from build123d import *

# Parameters (mm, degrees)
BOSS_EXTRUDE2_DEPTH = 22.86
CUT_EXTRUDE1_DEPTH  = 23.8600001
SKETCH10_R          = 3.96875
CUT_EXTRUDE2_DEPTH  = 23.8600001
BOSS_EXTRUDE4_DEPTH = 22.86
SKETCH13_R          = 3.96875
CUT_EXTRUDE5_DEPTH  = 23.8600001
LPATTERN1_COUNT     = 2
LPATTERN1_PITCH     = 64
SKETCH14_R          = 2.54
CUT_EXTRUDE6_DEPTH  = 23.8600001
SKETCH15_R          = 3.96875
CUT_EXTRUDE7_DEPTH  = 23.8600001
SKETCH16_R          = 3.96875
CUT_EXTRUDE8_DEPTH  = 23.8600001
SKETCH19_R          = 3.96875
CUT_EXTRUDE11_DEPTH = 23.8600001
SKETCH21_R          = 2.54
CUT_EXTRUDE12_DEPTH = 23.8600001
SKETCH23_R          = 4.16785984
SKETCH23_R_2        = 4.440390953
BOSS_EXTRUDE5_DEPTH = 22.86
CUT_EXTRUDE13_DEPTH = 23.8600001
FILLET1_R           = 3.175


with BuildPart() as part:
    # Sketch6 → Boss-Extrude2 (new body)
    with BuildSketch(Plane.XY):
        with BuildLine():
            Line((-68.006850091, -76.67090114), (-109.486767671, -48.656527855))
            Line((-109.486767671, -48.656527855), (-118.371760678, -61.812230963))
            Line((-118.371760678, -61.812230963), (18.447551645, -154.216158235))
            Line((18.447551645, -154.216158235), (135.729459338, 19.43912279))
            Line((135.729459338, 19.43912279), (-1.089852986, 111.843050063))
            Line((-1.089852986, 111.843050063), (-73.946795643, 3.966284577))
            Line((-73.946795643, 3.966284577), (-56.624438948, -7.732749433))
            ThreePointArc((-56.624438948, -7.732749433), (-43.058385537, 37.577891571), (0, 57.15))
            ThreePointArc((0, 57.15), (56.404848571, 31.095576642), (70.829334649, -29.338471048))
            add(Edge.make_bspline(
                [(70.829334649, -29.338471048), (70.811686062, -29.418295928), (70.776015112, -29.578104383), (70.713320217, -29.85478305), (70.619021771, -30.262929245), (70.501052001, -30.762086912), (70.364034474, -31.322191481), (70.199318515, -31.970958926), (70.000453855, -32.723919765), (69.795103485, -33.469783355), (69.582015398, -34.214296028), (69.361377803, -34.956693289), (69.133257682, -35.696762218), (68.838782679, -36.61892651), (68.470566207, -37.720710028), (68.019498024, -38.998776477), (67.474836154, -40.448808619), (66.901337925, -41.887676852), (66.299328392, -43.31485223), (65.669141732, -44.729810424), (65.011119088, -46.132040323), (64.325609411, -47.52103904), (63.612968547, -48.896314904), (62.87355937, -50.257385735), (62.107751613, -51.603779381), (61.315921169, -52.935034173), (60.49845004, -54.250698756), (59.655726138, -55.550331897), (58.571247582, -57.154294757), (57.220953058, -59.045283389), (55.576035723, -61.200397094), (53.604026134, -63.590264702), (51.54329346, -65.904053004), (49.39728314, -68.138962994), (47.169496434, -70.29235602), (44.863486103, -72.361752995), (42.482847363, -74.344831806), (40.031215607, -76.239428526), (36.882516177, -78.494556171), (32.976808929, -81.016011003), (28.250788286, -83.68089187), (21.41551215, -86.919136497), (14.30829026, -89.526654921), (6.996956895, -91.488176442), (-0.451922312, -92.797413176), (-6.61686174, -93.456358442), (-12.81195397, -93.702029749), (-19.009644204, -93.537285056), (-25.183124422, -92.966685286), (-31.306438312, -91.996382122), (-36.598524037, -90.804323442), (-41.072542301, -89.543185606), (-44.752319298, -88.33589156), (-47.664184976, -87.27761875), (-50.541347258, -86.128353728), (-53.381128552, -84.889612663), (-56.180924218, -83.562977818), (-58.593536599, -82.326710176), (-60.633378351, -81.214215821), (-62.313751085, -80.252471782), (-63.646071553, -79.462491566), (-64.966093336, -78.652178853), (-66.222359154, -77.854259082), (-67.143044791, -77.250601571), (-67.736251212, -76.85365602), (-68.006850091, -76.67090114)],
                knots=[0.071020771, 0.071020771, 0.071020771, 0.071020771, 0.071020771, 0.072848477, 0.074676184, 0.07650389, 0.078331597, 0.08198701, 0.085642423, 0.089297836, 0.092953249, 0.096608662, 0.100264075, 0.103919488, 0.107574901, 0.114885727, 0.122196554, 0.12950738, 0.136818214, 0.144129048, 0.151439882, 0.158750716, 0.166061558, 0.173372401, 0.180683243, 0.187994085, 0.195304924, 0.202615763, 0.209926602, 0.217237441, 0.231859103, 0.246480766, 0.261102426, 0.275724085, 0.290345754, 0.304967424, 0.319589099, 0.334210774, 0.348832457, 0.36345414, 0.392697464, 0.421940789, 0.451184112, 0.506140643, 0.535383973, 0.564627303, 0.593870641, 0.623113979, 0.652357319, 0.68160066, 0.710843985, 0.740087309, 0.754708984, 0.769330659, 0.783952333, 0.798574008, 0.813195669, 0.82781733, 0.842438991, 0.849749821, 0.857060652, 0.86437149, 0.871682327, 0.878993165, 0.885158103, 0.885158103, 0.885158103, 0.885158103, 0.885158103], degree=4))
        make_face()
    extrude(amount=BOSS_EXTRUDE2_DEPTH)

    # Sketch8 → Cut-Extrude1 (cut, through all)
    with BuildSketch(Plane.XY.offset(22.86)):
        Polygon((-71.011229489, -93.798205788), (-53.378672597, -90.381637707), (-42.854110111, -97.489632113), (-39.43754203, -115.122189004), align=None)
    extrude(amount=-CUT_EXTRUDE1_DEPTH, mode=Mode.SUBTRACT)

    # Sketch10 → Cut-Extrude2 (cut, through all)
    with BuildSketch(Plane.XY.offset(22.86)):
        with Locations((4.996496209, -84.796642912)):
            Circle(SKETCH10_R)
        with Locations((40.816310536, -31.759477627)):
            Circle(SKETCH10_R)
        with Locations((76.636124864, 21.277687659)):
            Circle(SKETCH10_R)
        with Locations((-45.295165913, -45.214466102)):
            Circle(SKETCH10_R)
    extrude(amount=-CUT_EXTRUDE2_DEPTH, mode=Mode.SUBTRACT)

    # Sketch12 → Boss-Extrude4 (add, through all)
    with BuildSketch(Plane.XY.offset(22.86)):
        Polygon((135.729459338, 19.43912279), (67.319803176, 65.641086427), (88.643786393, 97.214773886), (157.053442554, 51.01281025), align=None)
    extrude(amount=-BOSS_EXTRUDE4_DEPTH)

    # Sketch13 → Cut-Extrude5 (cut, through all)
    with BuildSketch(Plane.XY.offset(22.86)):
        with Locations((94.899221836, -29.671127724)):
            Circle(SKETCH13_R)
    cut_extrude5 = extrude(amount=-CUT_EXTRUDE5_DEPTH, mode=Mode.SUBTRACT)

    # LPattern1: Cut-Extrude5 ×2
    with Locations(*[Vector(-0.559684599, -0.828705708, 0) * (i * LPATTERN1_PITCH) for i in range(1, LPATTERN1_COUNT)]):
        add(cut_extrude5, mode=Mode.SUBTRACT)

    # Sketch14 → Cut-Extrude6 (cut, through all)
    with BuildSketch(Plane.XY.offset(22.86)):
        with Locations((71.72703343, -52.635713164)):
            Circle(SKETCH14_R)
        with Locations((35.907219102, -105.67287845)):
            Circle(SKETCH14_R)
        with Locations((115.740620068, 63.589229581)):
            Circle(SKETCH14_R)
    extrude(amount=-CUT_EXTRUDE6_DEPTH, mode=Mode.SUBTRACT)

    # Sketch15 → Cut-Extrude7 (cut, through all)
    with BuildSketch(Plane.XY.offset(22.86)):
        with Locations((-105.147343009, -59.249804902)):
            Circle(SKETCH15_R)
        with Locations((15.885125585, -140.991740566)):
            Circle(SKETCH15_R)
        with Locations((1.472573075, 98.618632394)):
            Circle(SKETCH15_R)
    extrude(amount=-CUT_EXTRUDE7_DEPTH, mode=Mode.SUBTRACT)

    # Sketch16 → Cut-Extrude8 (cut, through all)
    with BuildSketch(Plane.XY.offset(22.86)):
        with Locations((92.060354474, 79.582216994)):
            Circle(SKETCH16_R)
        with Locations((139.420885662, 47.596242169)):
            Circle(SKETCH16_R)
    extrude(amount=-CUT_EXTRUDE8_DEPTH, mode=Mode.SUBTRACT)

    # Sketch19 → Cut-Extrude11 (cut, through all)
    with BuildSketch(Plane.XY.offset(22.86)):
        with Locations((-65.680233685, -85.904783923)):
            Circle(SKETCH19_R)
    extrude(amount=-CUT_EXTRUDE11_DEPTH, mode=Mode.SUBTRACT)

    # Sketch21 → Cut-Extrude12 (cut, through all)
    with BuildSketch(Plane.XY.offset(22.86)):
        with Locations((-13.666272317, 70.530227577)):
            Circle(SKETCH21_R)
        with Locations((26.00698069, 78.217505758)):
            Circle(SKETCH21_R)
        with Locations((-86.729358658, -71.688795112)):
            Circle(SKETCH21_R)
        with Locations((-8.64928203, -120.590613931)):
            Circle(SKETCH21_R)
    extrude(amount=-CUT_EXTRUDE12_DEPTH, mode=Mode.SUBTRACT)

    # Sketch23 → Boss-Extrude5 (add, through all)
    with BuildSketch(Plane.XY.offset(22.86)):
        with Locations((-65.680233685, -85.904783923)):
            Circle(SKETCH23_R)
        with Locations((-86.729358658, -71.688795112)):
            Circle(SKETCH23_R_2)
    extrude(amount=-BOSS_EXTRUDE5_DEPTH)

    # Sketch25 → Cut-Extrude13 (cut, through all)
    with BuildSketch(Plane.XY.offset(22.86)):
        Polygon((85.800588631, 93.004948891), (87.167215863, 85.951926135), (71.529628171, 62.797888664), (67.319803176, 65.641086427), align=None)
    extrude(amount=-CUT_EXTRUDE13_DEPTH, mode=Mode.SUBTRACT)

    # Fillet1
    fillet1_edges = [part.edges().sort_by_distance(p)[0] for p in [
        (-73.946795643, 3.966284577, 11.43),
        (-1.089852986, 111.843050063, 11.43),
        (18.447551645, -154.216158235, 11.43),
        (-118.371760678, -61.812230963, 11.43),
        (-109.486767671, -48.656527855, 11.43),
        (85.800588631, 93.004948891, 11.43),
        (87.167215863, 85.951926135, 11.43),
        (71.529628171, 62.797888664, 11.43),
        (-39.43754203, -115.122189004, 11.43),
        (-71.011229489, -93.798205788, 11.43),
        (-53.378672597, -90.381637707, 11.43),
        (-42.854110111, -97.489632113, 11.43),
        (157.053442554, 51.01281025, 11.43),
        (88.643786393, 97.214773886, 11.43),
    ]]
    fillet(fillet1_edges, radius=FILLET1_R)


solid = part.part
Verification items for the finished model (mm, model axes). A direction names the side the tool comes from. Round coordinates to 2 decimals unless told otherwise and drop trailing zeros. Loops run counter-clockwise (first coordinate to the right, second up) from the corner with the lowest first, then second, coordinate; pieces in that order, holes last. Notation, with made-up numbers: (63, -10.75) - (99, -10.75) arc R23 ccw to (99, 21.25) - close; hole circle Ø7 at (-14.75, 19). An arc over 180 degrees is marked (long way). Answer in a Markdown table with one row per item. Add a question column.
Q1. Section check A-A on z = 5. State how many separate pieces and enclosed holes the cut face has, plus the area to 3 significant figures.
Q2. Material ranges on line 1 (Y direction, x = 17.5, z = 17.75); line 2 (Y direction, x = 37, z = 17.25); line 3 (X direction, y = -58, z = 4), recorded low to high.
Q3. Tool access check on faces 1 (the face through (-37.033, 58.623, 11.27)), 2 (the face through (-64.073, -2.702, 11.27)), 3 (the face through (55.83, 31.79, 11.27)). Record the directions out of +Z, -Z, +X, -X, +Y, -Y that give a thin tool (end or side, any length) a straight path to the whole face; none if there is none.
Q4. Release check for a two-part mould opening along X. For faces 4 (the face through (-62.3, -92.11, 11.59)), 5 (the face through (122.41, 74.41, 11.59)), 6 (the face through (81, -11, 0)), 7 (the face through (-94.226, -78.119, 11.27)) record: pulls with the +X half, pulls with the -X half, needs draft (parallel to the pull), parting line crosses it, or undercut.
Q5. Section check D-D on y = -17.5. Enter the section's corners in (x, z), plus the area to 3 significant figures.
Q6. Section check C-C on x = 132. Enter the section's corners in (y, z), plus the area to 3 significant figures.
Q7. Gauge pin test, flat ends, axial feed: pin 1 (8 mm diameter, centred on y = 61.5, z = 10, fed in from -X); pin 2 (4 mm diameter, centred on x = 26.01, y = 78.22, fed in from -Z); pin 3 (1 mm diameter, centred on x = 109.5, z = 17.5, fed in from +Y); pin 4 (8 mm diameter, centred on y = -47.5, z = 13.5, fed in from +X). Record the tip position at first contact, or that the pin passes through.
Found:
| question | item | result |
|---|---|---|
| 1 | separate pieces | 1 |
| 1 | enclosed holes | 14 |
| 1 | area | 18,000 mm² |
| 2 | line 1 | y = -152.98 to -144.62, -137.37 to -88.27, 55.31 to 99.29 |
| 2 | line 2 | y = -126.75 to -107.97, -103.38 to -78.37, 47.59 to 86.12 |
| 2 | line 3 | x = -115.8 to -108.91, -101.38 to -95.65, 57.96 to 83.43 |
| 3 | face 1 | +Z, -Z, -X, +Y |
| 3 | face 2 | +Z, -Z, -X |
| 3 | face 3 | +Z, -Z |
| 4 | face 4 | undercut |
| 4 | face 5 | pulls with the +X half |
| 4 | face 6 | needs draft |
| 4 | face 7 | pulls with the -X half |
| 5 | outline | (72.42, 0) - (110.78, 0) - (110.78, 22.86) - (72.42, 22.86) - close |
| 5 | area | 877 mm² |
| 6 | outline | (13.92, 0) - (67.93, 0) - (67.93, 22.86) - (13.92, 22.86) - close |
| 6 | area | 1,230 mm² |
| 7 | pin 1 | stops at x = -37.79 |
| 7 | pin 2 | passes through |
| 7 | pin 3 | stops at y = 83.47 |
| 7 | pin 4 | stops at x = 93.22 |
